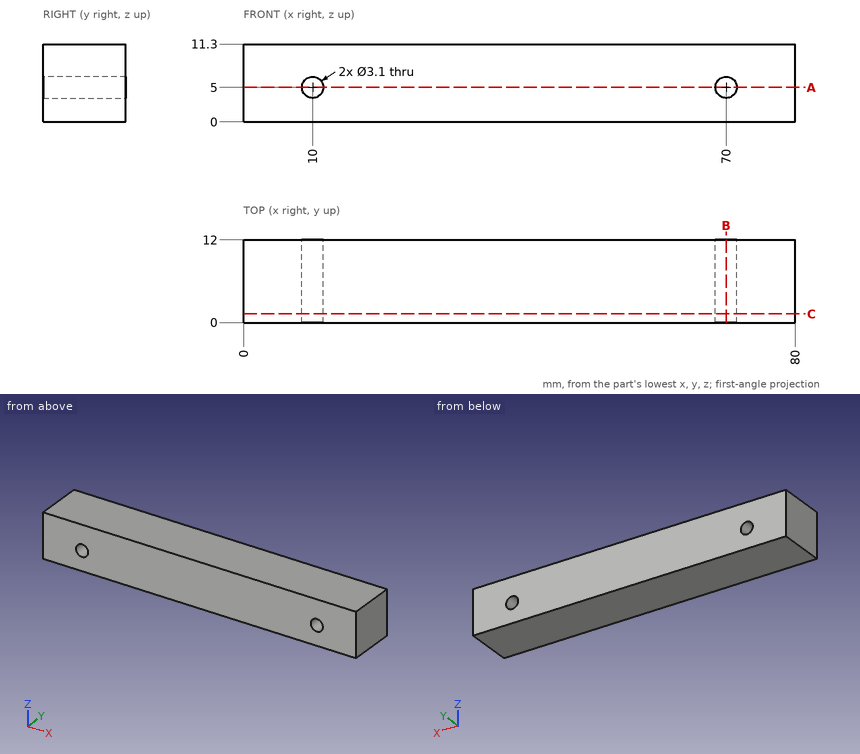
Can you work these out from the drawing? Everything is in mm from the part's minimum corner. Round coordinates to 2 decimals unless told otherwise and drop trailing zeros. Loops run counter-clockwise (first coordinate to the right, second up) from the corner with the lowest first, then second, coordinate; pieces in that order, holes last. Notation, with made-up numbers: (87.25, -27) - (107.25, -27) arc R28 cw to (107.25, -2) - close; hole circle Ø10 at (-0.5, 10). An arc over 180 degrees is marked (long way). Answer in a Markdown table with one row per item. Add a question column.
(1) I need wall thicknesses on line 1 along X through (y, z) = (3.75, 5); line 2 along Z through (x, y) = (70, 5.5); line 3 along X through (y, z) = (1.25, 6). Which ranges of each line are inside material? Lowest first, please.
(2) If we section it at B-B (x = 70): Please give me the cut outline in (y, z).
(3) I'm going to push a flat-ended pin straight in: pin 1 (4 mm diameter, centred on x = 10.5, y = 8, fed in from -Z). Where does the tip first touch, or does it pass through?
(4) If we section it at A-A (z = 5): Please give me the cut outline in (x, y).
(5) If we section it at C-C (y = 1.25): Please give me the cut outline in (x, z).
Model answer:
| question | item | result |
|---|---|---|
| 1 | line 1 | x = 0 to 8.45, 11.55 to 68.45, 71.55 to 80 |
| 1 | line 2 | z = 0 to 3.45, 6.55 to 11.3 |
| 1 | line 3 | x = 0 to 8.82, 11.18 to 68.82, 71.18 to 80 |
| 2 | outline | (0, 0) - (12, 0) - (12, 3.45) - (0, 3.45) - close; (0, 6.55) - (12, 6.55) - (12, 11.3) - (0, 11.3) - close |
| 3 | pin 1 | stops at z = 0 |
| 4 | outline | (0, 0) - (8.45, 0) - (8.45, 12) - (0, 12) - close; (11.55, 0) - (68.45, 0) - (68.45, 12) - (11.55, 12) - close; (71.55, 0) - (80, 0) - (80, 12) - (71.55, 12) - close |
| 5 | outline | (0, 0) - (80, 0) - (80, 11.3) - (0, 11.3) - close; hole circle Ø3.1 at (10, 5); hole circle Ø3.1 at (70, 5) |
